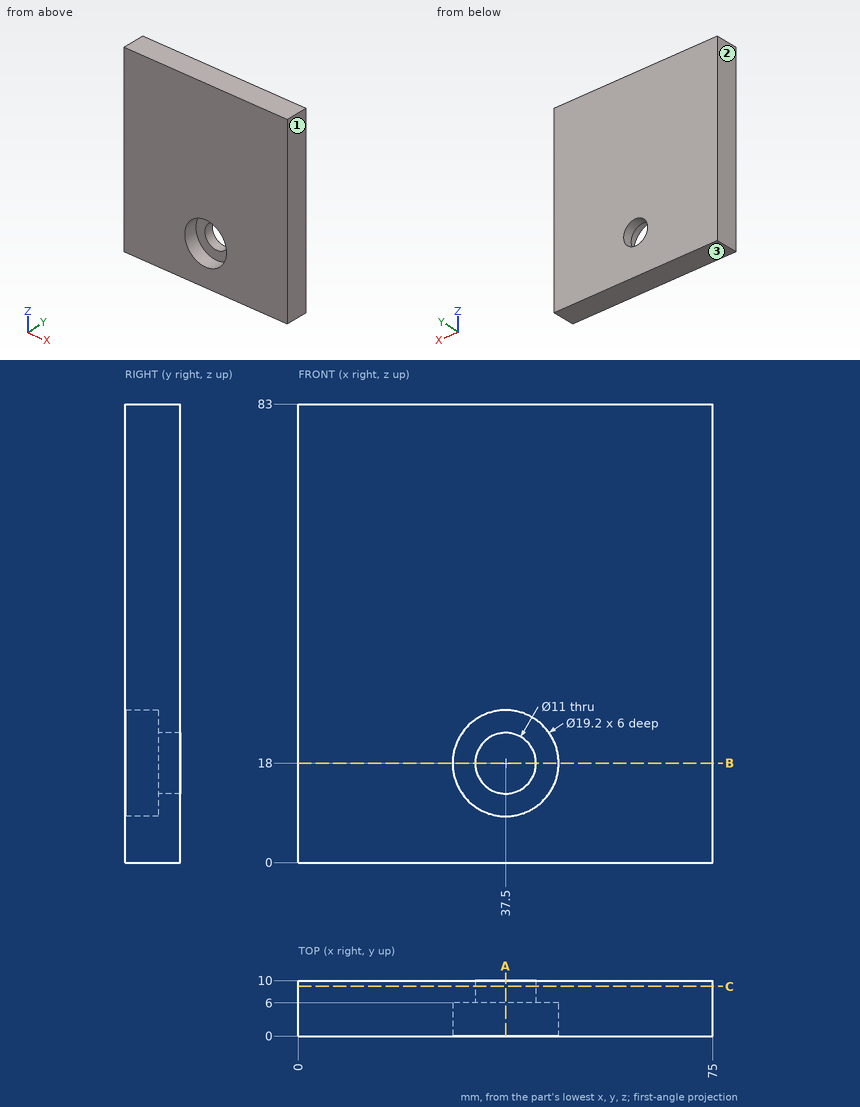
Can you work these out from the drawing? Everything is in mm from the part's minimum corner. Round coordinates to 2 decimals unless told otherwise and drop trailing zeros. Loops run counter-clockwise (first coordinate to the right, second up) from the corner with the lowest first, then second, coordinate; pieces in that order, holes last. Notation, with made-up numbers: (24, -10.75) -> (79, -10.75) arc R25 cw to (79, 4.25) -> close; hole circle Ø2 at (64, -16). An arc over 180 degrees is marked (long way). Put each result on its own line as item: value.
Q1. Thinking about a two-plate mould opening in X: for the marked faces 1, 2 and 3, which applies, pulls with the +X half, pulls with the -X half, needs draft (parallel to the pull), parting line crosses it, or undercut?
Checks:
face 1: pulls with the +X half
face 2: pulls with the -X half
face 3: needs draft
Q2. I want a section at C-C on y = 9. Write out the boundary of the cut face in (x, z), and give its area (3 significant figures).
Checks:
outline: (0, 0) -> (75, 0) -> (75, 83) -> (0, 83) -> close; hole circle Ø11 at (37.5, 18)
area: 6,130 mm2
Q3. Please list where these lines run through material, in increasing order: line 1 (Z direction, x = 37.5, y = 9.1); line 2 (Z direction, x = 37.5, y = 2); line 3 (X direction, y = 5.5, z = 25.5). Write a range as from..to.
Checks:
line 1: 0..12.5, 23.5..83
line 2: 0..8.4, 27.6..83
line 3: 0..31.51, 43.49..75
Q4. I want a section at A-A on x = 37.5. Write out the boundary of the cut face in (y, z).
Checks:
outline: (0, 0) -> (10, 0) -> (10, 12.5) -> (6, 12.5) -> (6, 8.4) -> (0, 8.4) -> close; (0, 27.6) -> (6, 27.6) -> (6, 23.5) -> (10, 23.5) -> (10, 83) -> (0, 83) -> close
Q5. I want a section at B-B on z = 18. Write out the boundary of the cut face in (x, y).
Checks:
outline: (0, 0) -> (27.9, 0) -> (27.9, 6) -> (32, 6) -> (32, 10) -> (0, 10) -> close; (43, 6) -> (47.1, 6) -> (47.1, 0) -> (75, 0) -> (75, 10) -> (43, 10) -> close
